The model under review builds one solid part; all positions refer to its coordinate system, in mm. A direction names the side the tool comes from. Round coordinates to 2 decimals unless told otherwise and drop trailing zeros. Loops run counter-clockwise (first coordinate to the right, second up) from the corner with the lowest first, then second, coordinate; pieces in that order, holes last. Notation, with made-up numbers: M -7,16.5 L 11,16.5 A19 cw 11,53.5 Z; hole C 4.5,-26.75 d8. An arc over 180 degrees is marked long. Return JSON: item names as keys, results as strings. Group by question number.
Q1. To check wall thickness, follow line 1 along X through (y, z) = (0, 54); line 2 along Y through (x, z) = (10, 32). State the ranges of each line that lie inside material, in increasing order.
Q2. For faces 1 (the face through (19.55, 8.36, 30.43)), 2 (the face through (0.26, -19.57, 0.45)), list the 3-axis set-ups (+Z, -Z, +X, -X, +Y, -Y) from which the entire face can be reached by the end or side of a thin tool; tool diameter is ignored.
Q3. Consider section D-D (z = 25). State the section outline as (x, y) points, and give its area (3 significant figures).
Q4. Consider section A-A (x = 10). State the section outline as (y, z) points, and give its area (3 significant figures).
Q5. Clearance check with flat-ended pins moving along their axes: pin 1 Ø5 at (x, y) = (1, 1) entering from +Z; pin 2 Ø3 at (x, y) = (10, 10) entering from -Z; pin 3 Ø9 at (y, z) = (7, 15) entering from +X; pin 4 Ø9 at (x, y) = (13, 5) entering from -Z. State where each tip first meets the part, or that it passes through.
Q6. Consider section C-C (z = 55.5). State the section outline as (x, y) points.
Solid Edge part; units mm, degrees
sketch "Sketch1" plane through (0, 0, 0) normal (0, 0, 1) x (1, 0, 0)
  line L0 (-20, -20) -> (20, -20)
  line L1 (20, -20) -> (20, 20)
  line L2 (20, 20) -> (-20, 20)
  line L3 (-20, 20) -> (-20, -20)
extrude "Protrusion1" add sketch "Sketch1" along normal blind 60
sketch "Sketch2" plane through (0, 0, 0) normal (0, 0, -1) x (0, 1, 0)
  line L0 (20, 20) -> (0, 20)
  line L1 (0, 20) -> (0, 0)
  line L2 (0, 0) -> (20, 0)
  line L3 (20, 0) -> (20, 20)
extrude "ExtrudedCutout_1" cut sketch "Sketch2" against normal blind 30
hole "Hole_3" at (10, 10, 60) direction (0, 0, -1) diameter 5 end up to next
hole "Hole_4" at (0, 0, 60) direction (0, 0, -1) diameter 10 depth 20
fillet "Round_1" radius 1.5 18 edges at (20, 20, 45) (-20, 20, 30) (20, -20, 30) (-20, -20, 30) (20, -10, 0) (0, -20, 0) (-20, 0, 0) (-10, 20, 0) (0, 20, 15) (0, 10, 0) (10, 0, 0) (20, 0, 15) (20, 10, 30) (10, 20, 30) (0, 20, 60) (-20, 0, 60) (20, 0, 60) (0, -20, 60)
properties material "Wood, Oak"
Values:
{
 "1": {"line 1": "x = -20 to -5, 5 to 20", "line 2": "y = -20 to 7.5, 12.5 to 20"},
 "2": {"face 1": "-Z, +X, +Y", "face 2": "-Z, +X, -X, -Y"},
 "3": {"outline": "M -20,-18.5 A1.5 ccw -18.5,-20 L 18.5,-20 A1.5 ccw 20,-18.5 L 20,-1.5 A1.5 ccw 18.5,0 L 0,0 L 0,18.5 A1.5 ccw -1.5,20 L -18.5,20 A1.5 ccw -20,18.5 Z", "area": "1,200 mm2"},
 "4": {"outline": "M -20,1.5 A1.5 ccw -18.5,0 L -1.5,0 A1.5 ccw 0,1.5 L 0,30 L 7.5,30 L 7.5,60 L -18.5,60 A1.5 ccw -20,58.5 Z; M 12.5,30 L 18.5,30 A1.5 ccw 20,31.5 L 20,58.5 A1.5 ccw 18.5,60 L 12.5,60 Z", "area": "1,650 mm2"},
 "5": {"pin 1": "stops at z = 40", "pin 2": "passes through", "pin 3": "stops at x = 0", "pin 4": "stops at z = 30"},
 "6": {"outline": "M -20,-18.5 A1.5 ccw -18.5,-20 L 18.5,-20 A1.5 ccw 20,-18.5 L 20,18.5 A1.5 ccw 18.5,20 L -18.5,20 A1.5 ccw -20,18.5 Z; hole C 0,0 d10; hole C 10,10 d5"}
}
